The model under review builds one solid part; all positions refer to its coordinate system, in mm. A direction names the side the tool comes from. Round coordinates to 2 decimals unless told otherwise and drop trailing zeros. Loops run counter-clockwise (first coordinate to the right, second up) from the corner with the lowest first, then second, coordinate; pieces in that order, holes last. Notation, with made-up numbers: (24.5, 38.25) -> (60.5, 38.25) arc R17 cw to (60.5, 48.25) -> close; hole circle Ø8 at (8, 30). An arc over 180 degrees is marked (long way). Use a Markdown table: item, result. Add a question column.
1) Insertion check: pin 1 (3 mm diameter, centred on x = -0.5, y = -1, fed in from -Z); pin 2 (2 mm diameter, centred on y = -2, z = 23.5, fed in from +X); pin 3 (2 mm diameter, centred on y = -3, z = 10.5, fed in from -X); pin 4 (1.5 mm diameter, centred on x = -1, z = 4.5, fed in from -Y) (3 decimals). Each pin has a flat end and moves straight along its axis. Give the tip position at first contact, or say it passes through.
2) Wall thickness on probe 1 along Y at (x, z) = (0, 6); probe 2 along Z at (x, y) = (0.5, -2.75); probe 3 along Z at (x, y) = (3.25, 1): over which ranges is each line inside the solid? List them lowest first.
3) For faces 4 (the cylindrical face through (-0.661, 5.037, 30.444)), 5 (the cylindrical face through (0.248, -1.116, 3.882)), list the 3-axis set-ups (+Z, -Z, +X, -X, +Y, -Y) from which the entire face can be reached by the end or side of a thin tool; tool diameter is ignored.
4) Mouldability with a two-part tool opening along Y and no side actions: class faces 1 (the cylindrical face through (-0.258, 1.964, 3.882)), 2 (the flat face through (-0.1, -3.3, 27.94)), 3 (the flat face through (0, 0, 7.874)) as released by +Y, released by -Y, zero draft, split by the parting line, or undercut.
5) Consider section B-B on z = 3. Give the boundary of the cut face in (x, y).
6) Consider section D-D on z = 19. Give the boundary of the cut face in (x, y).
7) Consider section A-A on y = 0. Give the boundary of the cut face in (x, z), plus the area to 3 significant figures.
from build123d import *

# Parameters (mm, degrees)
SKETCH1_R           = 1.9808444
BOSS_EXTRUDE1_DEPTH = 7.874
SKETCH2_R           = 1.143
CUT_EXTRUDE2_DEPTH  = 8.874
SKETCH3_R           = 2.99147738
BOSS_EXTRUDE2_DEPTH = 20.066
SKETCH4_R           = 5.08
BOSS_EXTRUDE3_DEPTH = 5.08


with BuildPart() as part:
    # Sketch1 → Boss-Extrude1 (new body)
    with BuildSketch(Plane.XY):
        Circle(SKETCH1_R)
    extrude(amount=BOSS_EXTRUDE1_DEPTH)

    # Sketch2 → Cut-Extrude2 (cut, through all)
    with BuildSketch(Plane(origin=(0, 0, 0), x_dir=(-1, 0, 0), z_dir=(0, 0, -1))):
        Circle(SKETCH2_R)
    extrude(amount=-CUT_EXTRUDE2_DEPTH, mode=Mode.SUBTRACT)

    # Sketch3 → Boss-Extrude2 (add)
    with BuildSketch(Plane.XY.offset(7.874)):
        Circle(SKETCH3_R)
    extrude(amount=BOSS_EXTRUDE2_DEPTH)

    # Sketch4 → Boss-Extrude3 (add)
    with BuildSketch(Plane.XY.offset(27.94)):
        Circle(SKETCH4_R)
    extrude(amount=BOSS_EXTRUDE3_DEPTH)


solid = part.part
Result set:
| question | item | result |
|---|---|---|
| 1 | pin 1 | z = 0 |
| 1 | pin 2 | x = 2.82 |
| 1 | pin 3 | x = -2.22 |
| 1 | pin 4 | y = -1.965 |
| 2 | probe 1 | -1.98 to -1.14, 1.14 to 1.98 |
| 2 | probe 2 | 7.87 to 33.02 |
| 2 | probe 3 | 27.94 to 33.02 |
| 3 | face 4 | +Z, -Z |
| 3 | face 5 | -Z |
| 4 | face 1 | split by the parting line |
| 4 | face 2 | zero draft |
| 4 | face 3 | undercut |
| 5 | outline | circle Ø3.96 at (0, 0); hole circle Ø2.29 at (0, 0) |
| 6 | outline | circle Ø5.98 at (0, 0) |
| 7 | outline | (-5.08, 27.94) -> (-2.99, 27.94) -> (-2.99, 7.87) -> (-1.98, 7.87) -> (-1.98, 0) -> (-1.14, 0) -> (-1.14, 7.87) -> (1.14, 7.87) -> (1.14, 0) -> (1.98, 0) -> (1.98, 7.87) -> (2.99, 7.87) -> (2.99, 27.94) -> (5.08, 27.94) -> (5.08, 33.02) -> (-5.08, 33.02) -> close |
| 7 | area | 185 mm2 |
